Geometry: see drawing. Coordinates: mm, zero at the bounding-box minimum. A direction names the side the tool comes from. Give positions to 0.01 mm unless a question says otherwise; leave off trailing zeros. Write each loop counter-clockwise with the first axis right and the second up, starting at its lowest first coordinate (ties: lowest second). Pieces come first, ordered by that corner, then holes. Notation, with made-up numbers: (32.5, -0.75) - (81.5, -0.75) arc R16 ccw to (81.5, 4.25) - close; hole circle Ø6 at (-33.75, 82.25). An arc over 180 degrees is marked (long way). Use CSV: the item, a comma, the result in double quotes. Start each with the question number.
(1) Draft query along X for the marked faces 4, 5 and 6. Return one class per face: released by +X, released by -X, zero draft, split by the parting line, or undercut.
(2) Section B-B on z = 11. Count the separate pieces of the cut face and the enclosed holes in it, and give its area (3 significant figures).
(3) Section A-A on x = 20. Output: boundary loops of the cut face in (y, z).
(4) Reachability of the marked faces 1, 2 and 3 from +Z, -Z, +X, -X, +Y, -Y: full face, straight path, thin tool, end or side. Return the list, or none.
(5) First-contact query: pin 1 Ø5 at (x, z) = (86.5, 21) entering from -Y; pin 2 Ø10 at (x, z) = (22, 37.5) entering from +Y; pin 3 Ø22 at (x, z) = (80, 33) entering from -Y. Flat tips, straight axial feed; report the tip coordinate or a pass-through.
(6) Line query: probe 1 along Z at (x, y) = (65, 53.4); probe 2 along Z at (x, y) = (50, 6); probe 3 along Y at (x, z) = (75, 12.5). Output: solid intervals per line, ascending. Write a range as [from, to].
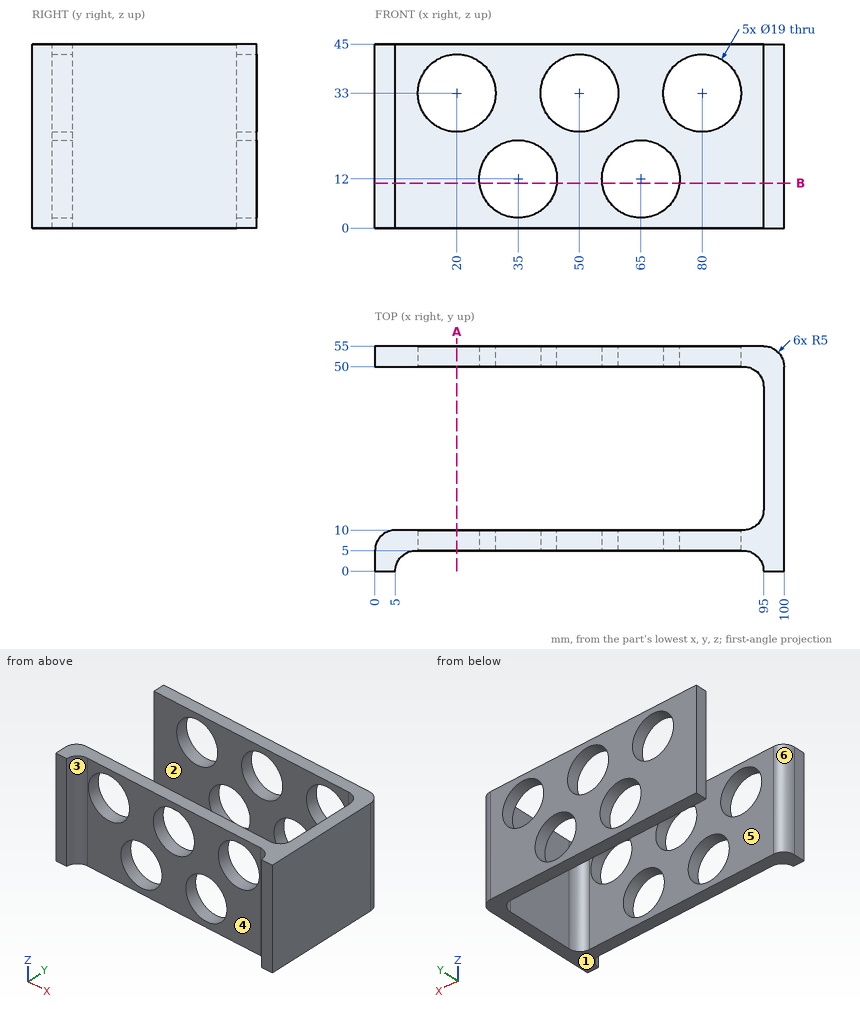
Check values:
1,face 4,"undercut"
1,face 5,"zero draft"
1,face 6,"released by -X"
2,separate pieces,"5"
2,enclosed holes,"0"
2,area,"883 mm²"
3,outline,"(5, 0) - (10, 0) - (10, 23.5) - (5, 23.5) - close; (5, 42.5) - (10, 42.5) - (10, 45) - (5, 45) - close; (50, 0) - (55, 0) - (55, 23.5) - (50, 23.5) - close; (50, 42.5) - (55, 42.5) - (55, 45) - (50, 45) - close"
4,face 1,"-Z, +X, -X, +Y, -Y"
4,face 2,"+Z, -Z, -X"
4,face 3,"+Z, -Z, -Y"
5,pin 1,"stops at y = 5"
5,pin 2,"stops at y = 55"
5,pin 3,"stops at y = 4.9"
6,probe 1,"z = [0, 2.5], [21.5, 45]"
6,probe 2,"z = [0, 23.5], [42.5, 45]"
6,probe 3,"y = [5, 10], [50, 55]"
